The listing builds one solid part. Answer for the finished solid, in the listing's coordinates (mm). Face numbers are marked on the shaded views. A direction names the side the tool comes from. Round coordinates to 2 decimals unless told otherwise and drop trailing zeros. Order: outer loops, then holes, each group sorted by start corner. A loop starts at its lowest first (then second) coordinate and runs counter-clockwise, first axis right, second up. Notation, with made-up numbers: M 41.5,79 L 61.5,79 A36 ccw 61.5,114 Z; hole C 77.25,64.5 d2. An arc over 180 degrees is marked long. Write item = value, one per line. Start each with the question number.
(1) Which of the six approach directions +Z, -Z, +X, -X, +Y, -Y give full straight-line access (tool end or side, diameter ignored) to the marked faces 4, 5, 6 and 7?
(2) A cutting plane is placed at C-C, the plane z = -7. Determine the outline of the cut face in (x, y), and give its area (3 significant figures).
(3) A cutting plane is placed at A-A, the plane y = 24.5. Determine the outline of the cut face in (x, z).
(4) Straight lines are drawn through the part: probe 1 along X at (y, z) = (1, -7); probe 2 along X at (y, z) = (25.5, 0.5); probe 3 along X at (y, z) = (7.5, 17). For each, find the intervals that lie inside material, in ascending order. Write a range as from..to.
(5) Each of these flat-tipped pins is pushed along its axis until it touches: pin 1 (4 mm diameter, centred on x = 25, y = 21, fed in from +Z); pin 2 (4 mm diameter, centred on x = 12.5, z = 15.5, fed in from +Y); pin 3 (8 mm diameter, centred on x = 27.5, y = 38.5, fed in from -Z); pin 4 (3.5 mm diameter, centred on y = 24, z = -3, fed in from -X). Where does it stop, or does it pass through?
(6) A cutting plane is placed at D-D, the plane z = 6.5. Determine the outline of the cut face in (x, y).
(7) A cutting plane is placed at B-B, the plane x = 12.5. Determine the outline of the cut face in (y, z).
(8) For a pull along X with two mould halves and no side action, classify the marked faces 1, 2 and 3 as released by +X, released by -X, zero draft, split by the parting line, or undercut.
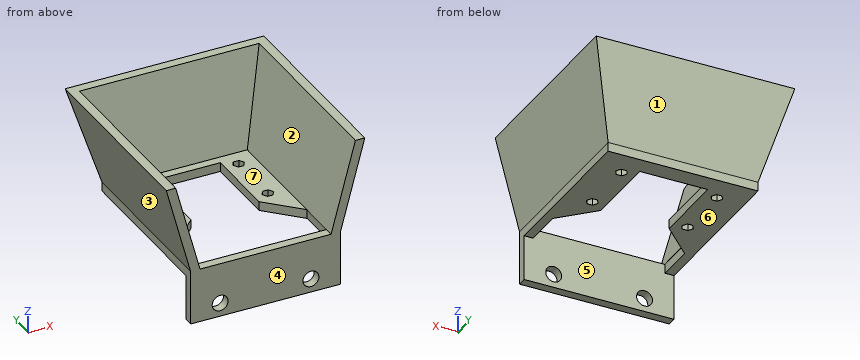
from build123d import *

# Parameters (mm, degrees)
BOSS_EXTRUDE1_DEPTH = 2
SKETCH2_W           = 33
SKETCH2_H           = 38
BOSS_EXTRUDE2_DEPTH = 20
BOSS_EXTRUDE2_DRAFT = -15
SHELL1_T            = -2
SKETCH3_W           = 33
SKETCH3_H           = 12
BOSS_EXTRUDE3_DEPTH = 2
SKETCH4_R           = 1.75
CUT_EXTRUDE1_DEPTH  = 61.547313622
SKETCH5_W           = 43.717967698
SKETCH5_H           = 20
CUT_EXTRUDE2_DEPTH  = 62.93071227


with BuildPart() as part:
    # Sketch1 → Boss-Extrude1 (new body)
    with BuildSketch(Plane.XY):
        Polygon((0, 0), (0, 38), (33, 38), (33, 0), (31, 0), (31, 10.417468245), (24, 17.417468245), (24, 34), (9, 34), (9, 17.417468245), (2, 10.417468245), (2, 0), align=None)
        Polygon((7.25, 32), (6.625, 33.082531755), (5.375, 33.082531755), (4.75, 32), (5.375, 30.917468245), (6.625, 30.917468245), align=None, mode=Mode.SUBTRACT)
        Polygon((7.25, 19.5), (6.625, 20.582531755), (5.375, 20.582531755), (4.75, 19.5), (5.375, 18.417468245), (6.625, 18.417468245), align=None, mode=Mode.SUBTRACT)
        Polygon((25.75, 19.5), (26.375, 18.417468245), (27.625, 18.417468245), (28.25, 19.5), (27.625, 20.582531755), (26.375, 20.582531755), align=None, mode=Mode.SUBTRACT)
        Polygon((28.25, 32), (27.625, 33.082531755), (26.375, 33.082531755), (25.75, 32), (26.375, 30.917468245), (27.625, 30.917468245), align=None, mode=Mode.SUBTRACT)
    extrude(amount=BOSS_EXTRUDE1_DEPTH)

    # Sketch3 → Boss-Extrude3 (add)
    with BuildSketch(Plane.XZ):
        with Locations((16.5, -4)):
            Rectangle(SKETCH3_W, SKETCH3_H)
    extrude(amount=-BOSS_EXTRUDE3_DEPTH)

    # Sketch4 → Cut-Extrude1 (cut, through all)
    with BuildSketch(Plane(origin=(0, 2, 0), x_dir=(1, 0, 0), z_dir=(0, 1, 0))):
        with Locations(Location((26.5, 7, 0), (0, 0, 270))):
            Circle(SKETCH4_R)
        with Locations(Location((6.5, 7, 0), (0, 0, 270))):
            Circle(SKETCH4_R)
    extrude(amount=-CUT_EXTRUDE1_DEPTH, mode=Mode.SUBTRACT)


with BuildPart() as body_2:
    # Sketch2 → Boss-Extrude2 (with draft: the straight prism first)
    with BuildSketch(Plane.XY.offset(2)):
        with Locations((16.5, 19)):
            Rectangle(SKETCH2_W, SKETCH2_H)
    extrude(amount=BOSS_EXTRUDE2_DEPTH)
    # Boss-Extrude2: the draft: its side faces are tilted about the plane it starts from
    boss_extrude2_sides = [body_2.faces().sort_by_distance(p)[0] for p in [
        (33, 19, 12),
        (16.5, 38, 12),
        (0, 19, 12),
        (16.5, 0, 12),
    ]]
    draft(boss_extrude2_sides, Plane.XY.offset(2), BOSS_EXTRUDE2_DRAFT)

    # Shell1
    shell1_openings = [body_2.faces().sort_by_distance(p)[0] for p in [
        (16.5, 19, 22),
        (16.5, 19, 2),
        (16.5, -2.804272376, 12.465686984),
    ]]
    offset(amount=SHELL1_T, openings=shell1_openings, kind=Kind.INTERSECTION)

    # Sketch5 → Cut-Extrude2 (cut, through all)
    with BuildSketch(Plane.XZ):
        with Locations((16.5, 12)):
            Rectangle(SKETCH5_W, SKETCH5_H)
    extrude(amount=CUT_EXTRUDE2_DEPTH, mode=Mode.SUBTRACT)

    # Combine1: union part
    add(part.part)


solid = body_2.part
Reported:
q1.face_4 = +Z, -Z, +X, -X, -Y
q1.face_5 = -Z
q1.face_6 = -Z, +X, -X, +Y
q1.face_7 = +Z, -Y
q2.outline = M 0,0 L 4.75,0 L 4.75,2 L 0,2 Z; M 8.25,0 L 24.75,0 L 24.75,2 L 8.25,2 Z; M 28.25,0 L 33,0 L 33,2 L 28.25,2 Z
q2.area = 52.0 mm²
q3.outline = M -5.36,22 L 0,2 L 0,0 L 9,0 L 9,2 L 2.07,2 L -3.29,22 Z; M 24,0 L 33,0 L 33,2 L 38.36,22 L 36.29,22 L 30.93,2 L 24,2 Z
q4.probe_1 = 0..4.75, 8.25..24.75, 28.25..33
q4.probe_2 = 0..9, 24..33
q4.probe_3 = -4.02..-1.95, 34.95..37.02
q5.pin_1 = 2
q5.pin_2 = 42.15
q5.pin_3 = 0
q5.pin_4 = through
q6.outline = M -1.21,0 L 0.86,0 L 0.86,37.14 L 32.14,37.14 L 32.14,0 L 34.21,0 L 34.21,39.21 L -1.21,39.21 Z
q7.outline = M 0,-10 L 2,-10 L 2,2 L 0,2 Z; M 34,0 L 38,0 L 38,2 L 43.36,22 L 41.29,22 L 35.93,2 L 34,2 Z
q8.face_1 = zero draft
q8.face_2 = undercut
q8.face_3 = released by -X
